```python
from build123d import *

# Parameters (mm, degrees)
BOSS_EXTRUDE1_DEPTH = 8
BOSS_EXTRUDE2_DEPTH = 11
BOSS_EXTRUDE3_DEPTH = 11
SKETCH5_R           = 1
CUT_EXTRUDE2_DEPTH  = 4
CUT_EXTRUDE1_REACH  = 13.565
SKETCH4_R           = 3


with BuildPart() as part:
    # Sketch1 → Boss-Extrude1 (new body)
    with BuildSketch(Plane.XY):
        Polygon((0, 0), (-7.250462296, 3.380946094), (-3.869516202, 10.63140839), (3.380946094, 7.250462296), align=None)
    extrude(amount=BOSS_EXTRUDE1_DEPTH)

    # Sketch2 → Boss-Extrude2 (add)
    with BuildSketch(Plane.XY.offset(8)):
        Polygon((-6.038297133, 2.815704195), (1.312984429, 2.815704195), (3.380946094, 7.250462296), (2.16878093, 7.815704195), (-5.182500632, 7.815704195), (-7.250462296, 3.380946094), align=None)
    extrude(amount=BOSS_EXTRUDE2_DEPTH)

    # Sketch3 → Boss-Extrude3 (add)
    with BuildSketch(Plane.XY.offset(8)):
        Polygon((-5.182500632, 7.815704195), (-8.434758101, 7.815704195), (-8.434758101, 2.815704195), (-6.038297133, 2.815704195), (-7.250462296, 3.380946094), align=None)
        Polygon((1.312984429, 2.815704195), (4.565241899, 2.815704195), (4.565241899, 7.815704195), (2.16878093, 7.815704195), (3.380946094, 7.250462296), align=None)
    extrude(amount=BOSS_EXTRUDE3_DEPTH)

    # Sketch5 → Cut-Extrude2 (cut)
    with BuildSketch(Plane(origin=(0, 0, 0), x_dir=(-1, 0, 0), z_dir=(0, 0, -1))):
        with Locations((1.934758101, 5.315704195)):
            Circle(SKETCH5_R)
    extrude(amount=-CUT_EXTRUDE2_DEPTH, mode=Mode.SUBTRACT)

    # Mirror2: part across face


with BuildPart() as part_1:
    add(part.part)
    add(part.part.mirror(Plane(origin=(-1.934758101, 5.315704195, 19), x_dir=(1, 0, 0), z_dir=(0, 0, 1))))

    # Sketch4 → Cut-Extrude1 (cut, up to next)
    with BuildSketch(Plane(origin=(3.380946094, 7.250462296, 0), x_dir=(0.906307787, -0.422618262, 0), z_dir=(0.422618262, 0.906307787, 0)), mode=Mode.PRIVATE) as cut_extrude1_sk1:
        with Locations((-4, -4)):
            Circle(SKETCH4_R)
    cut_extrude1_tool1 = extrude(cut_extrude1_sk1.sketch, amount=-CUT_EXTRUDE1_REACH, mode=Mode.PRIVATE) & part_1.part
    add(cut_extrude1_tool1.solids().sort_by_distance((-0.244285, 8.940935, 4))[0], mode=Mode.SUBTRACT)
    # Sketch4 → Cut-Extrude1 (cut, up to next)
    with BuildSketch(Plane(origin=(3.380946094, 7.250462296, 0), x_dir=(0.906307787, -0.422618262, 0), z_dir=(0.422618262, 0.906307787, 0)), mode=Mode.PRIVATE) as cut_extrude1_sk2:
        with Locations((-4, -34)):
            Circle(SKETCH4_R)
    cut_extrude1_tool2 = extrude(cut_extrude1_sk2.sketch, amount=-CUT_EXTRUDE1_REACH, mode=Mode.PRIVATE) & part_1.part
    add(cut_extrude1_tool2.solids().sort_by_distance((-0.244285, 8.940935, 34))[0], mode=Mode.SUBTRACT)


solid = part_1.part
```
The model under review builds one solid part; all positions refer to its coordinate system, in mm. A direction names the side the tool comes from. Give positions to 0.01 mm unless a question says otherwise; leave off trailing zeros. Write each loop counter-clockwise with the first axis right and the second up, starting at its lowest first coordinate (ties: lowest second). Pieces come first, ordered by that corner, then holes. Notation, with made-up numbers: M 17.25,-32.5 L 45.25,-32.5 A14 ccw 45.25,-12.5 Z; hole C 25,84.25 d1. An arc over 180 degrees is marked long. Write item = value, one per line. Start each with the question number.
Q1. Clearance check with flat-ended pins moving along their axes: pin 1 (2 mm diameter, centred on y = 9, z = 26, fed in from +X) (3 decimals); pin 2 (1.2 mm diameter, centred on x = -1.93, y = 5.32, fed in from -Z); pin 3 (3 mm diameter, centred on x = -6, z = 18.5, fed in from +Y). State where each tip first meets the part, or that it passes through.
Q2. Machinability: for faces 4 (the face through (-6, 2.8, 2.2)), 5 (the face through (-2, 9, 30)), 6 (the face through (-2, 2.816, 19)), which of the approach directions +Z, -Z, +X, -X, +Y, -Y give a long, thin tool a straight path to every point of the face, cutting with its end or side? Answer none if there is none.
Q3. We need section C-C (z = 18). State the section outline as (x, y) points, plus the area to 3 significant figures.
Q4. We need section B-B (x = -1.75). Give the number of separate pieces and of enclosed holes in the cut face, plus the area to 3 significant figures.
Q5. Mouldability with a two-part tool opening along Y and no side actions: class faces 1 (the face through (-2.71, 10.09, 5.72)), 2 (the face through (-6, 2.8, 35.8)), 3 (the face through (-1.198, 5.992, 37.422)) as released by +Y, released by -Y, zero draft, split by the parting line, or undercut.
Q6. For line 1 (Z direction, x = -1.75, y = 9.5); line 2 (Z direction, x = -4.75, y = 3); line 3 (Z direction, x = 0.25, y = 4), list the stretches that pass through material, from the lowest coordinate up.
Q7. We need section A-A (z = 32). State the section outline as (x, y) points.
Result set:
q1.pin_1 = through
q1.pin_2 = 6.94
q1.pin_3 = 7.82
q2.face_4 = -Z, -X, -Y
q2.face_5 = +X, -X, +Y
q2.face_6 = +X, -X, -Y
q3.outline = M -8.43,2.82 L 4.57,2.82 L 4.57,7.82 L -8.43,7.82 Z
q3.area = 65.0 mm2
q4.separate_pieces = 5
q4.enclosed_holes = 0
q4.area = 149 mm2
q5.face_1 = released by +Y
q5.face_2 = released by -Y
q5.face_3 = undercut
q6.line_1 = 0 to 1.46, 6.54 to 8, 30 to 31.46, 36.54 to 38
q6.line_2 = 0 to 1.45, 6.55 to 31.45, 36.55 to 38
q6.line_3 = 0 to 2.4, 5.6 to 32.4, 35.6 to 38
q7.outline = M -7.25,3.38 L -5.65,2.64 L -2.27,9.89 L -3.87,10.63 Z; M -1.6,0.75 L 0,0 L 3.38,7.25 L 1.78,8 Z
